The model under review builds one solid part; all positions refer to its coordinate system, in mm. A direction names the side the tool comes from. Round coordinates to 2 decimals unless told otherwise and drop trailing zeros. Write each loop counter-clockwise with the first axis right and the second up, starting at its lowest first coordinate (ties: lowest second). Pieces come first, ordered by that corner, then holes. Notation, with made-up numbers: (64.5, 48) - (69.5, 48) arc R25 ccw to (69.5, 73) - close; hole circle Ø2 at (-26.75, 58). An arc over 180 degrees is marked (long way). Return JSON: item names as keys, results as strings.
from build123d import *

# Parameters (mm, degrees)
F0_W     = 60
F0_H     = 38
F1_DEPTH = 36
F2_W     = 8
F2_H     = 15
F3_DEPTH = 15
F4_DEPTH = 28
F2_W_2   = 30
F2_H_2   = 18
F5_DEPTH = 36.001
F2_W_3   = 35
F2_H_3   = 8
F6_DEPTH = 10
F8_DEPTH = 8.001


with BuildPart() as f1:
    # F0 (on Front) → F1 (new body)
    with BuildSketch(Plane.XZ):
        Rectangle(F0_W, F0_H)
    extrude(amount=F1_DEPTH)

    # F2 (on face) → F3 (cut)
    with BuildSketch(Plane.XZ.offset(36)):
        with Locations((26, -3.5)):
            Rectangle(F2_W, F2_H)
    extrude(amount=-F3_DEPTH, mode=Mode.SUBTRACT)

    # F2 (on face) → F4 (cut)
    with BuildSketch(Plane.XZ.offset(36)):
        Polygon((0, -19), (22, -19), (22, -11), (22, 4), (22, 11), (10, 11), (-25, 11), (-30, 11), (-30, -1), (0, -1), align=None)
    extrude(amount=-F4_DEPTH, mode=Mode.SUBTRACT)

    # F2 (on face) → F5 (cut, through all)
    with BuildSketch(Plane.XZ.offset(36)):
        with Locations((-15, -10)):
            Rectangle(F2_W_2, F2_H_2)
    extrude(amount=-F5_DEPTH, mode=Mode.SUBTRACT)

    # F2 (on face) → F6 (cut)
    with BuildSketch(Plane.XZ.offset(36)):
        with Locations((-7.5, 15)):
            Rectangle(F2_W_3, F2_H_3)
    extrude(amount=-F6_DEPTH, mode=Mode.SUBTRACT)

    # F7 (on face) → F8 (cut, through all)
    with BuildSketch(Plane(origin=(0, 0, 11), x_dir=(1, 0, 0), z_dir=(0, 0, -1))):
        Polygon((-25, 26), (-7.5, 12.67333), (10, 26), align=None)
    extrude(amount=-F8_DEPTH, mode=Mode.SUBTRACT)


solid = f1.part
(1) Add section D-D (x = 21). Write out the cut boundary in (y, z).
Filled in:
{"outline": "(-36, 11) - (-8, 11) - (-8, -19) - (0, -19) - (0, 19) - (-36, 19) - close"}
(2) Add section A-A (y = -24.5). Write out the cut boundary in (x, z), plus the area to 3 significant figures.
Filled in:
{"outline": "(-30, 11) - (-23.03, 11) - (-23.03, 19) - (-30, 19) - close; (8.03, 11) - (22, 11) - (22, 4) - (30, 4) - (30, 19) - (8.03, 19) - close; (22, -19) - (30, -19) - (30, -11) - (22, -11) - close", "area": "352 mm2"}
(3) Wall thickness on line 1 (Z direction, x = 24, y = -27.5); line 2 (X direction, y = -13, z = -11); line 3 (Y direction, x = 8.5, z = 0.5): over which ranges is each line inside the solid? List them lowest first.
Filled in:
{"line 1": "z = -19 to -11, 4 to 19", "line 2": "x = 22 to 30", "line 3": "y = -8 to 0"}
(4) Add section B-B (z = -16.5). Write out the cut boundary in (x, y), plus the area to 3 significant figures.
Filled in:
{"outline": "(0, -8) - (22, -8) - (22, -36) - (30, -36) - (30, 0) - (0, 0) - close", "area": "464 mm2"}
(5) For faces 4 (the flat face through (26, -29, -11)), 5 (the flat face through (-16.37, -19.43, 14.94)), 6 (the flat face through (1, -8, 0)), list the 3-axis set-ups (+Z, -Z, +X, -X, +Y, -Y) from which the entire face can be reached by the end or side of a thin tool; tool diameter is ignored.
Filled in:
{"face 4": "+X, -X, -Y", "face 5": "+Z, -Z, -Y", "face 6": "-Z, -X, -Y"}
(6) Clearance check with flat-ended pins moving along their axes: pin 1 Ø14 at (y, z) = (-18, -9) entering from -X; pin 2 Ø9 at (x, z) = (-1.5, -8.5) entering from -Y; pin 3 Ø8.5 at (x, y) = (-3.5, -24.5) entering from -Z; pin 4 Ø10 at (x, y) = (7.5, -17) entering from -Z. State where each tip first meets the part, or that it passes through.
Filled in:
{"pin 1": "stops at x = 22", "pin 2": "stops at y = -8", "pin 3": "passes through", "pin 4": "stops at z = 11"}
(7) Add section C-C (y = -14.5). Write out the cut boundary in (x, z), plus the area to 3 significant figures.
Filled in:
{"outline": "(-30, 11) - (-9.9, 11) - (-9.9, 19) - (-30, 19) - close; (-5.1, 11) - (22, 11) - (22, -19) - (30, -19) - (30, 19) - (-5.1, 19) - close", "area": "682 mm2"}
(8) Mouldability with a two-part tool opening along Z and no side actions: class faces 1 (the flat face through (-15, -4, -1)), 2 (the flat face through (26, -29, 4)), 3 (the flat face through (0, -4, -10)) as released by +Z, released by -Z, zero draft, split by the parting line, or undercut.
Filled in:
{"face 1": "released by -Z", "face 2": "undercut", "face 3": "zero draft"}
